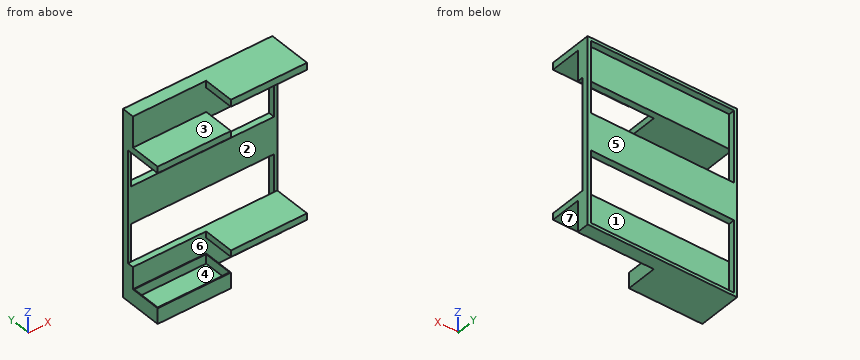
```python
from build123d import *

# Parameters (mm, degrees)
F0_W      = 609.6
F0_H      = 762
F0_W_2    = 584.5253169537
F0_H_2    = 736.8236780167
F1_DEPTH  = 25.4
F2_W      = 584.5253169537
F2_H      = 140.0518767754
F3_DEPTH  = 25.4
F4_W      = 609.6
F4_H      = 152.9776729027
F5_DEPTH  = 25.4
F6_W      = 607.6588928699
F6_H      = 151.1828005314
F7_DEPTH  = 25.4
F8_W      = 310.3615156889
F8_H      = 26.3459533453
F9_DEPTH  = 127
F10_W     = 299.2384843111
F10_H     = 25.4
F11_DEPTH = 127
F12_W     = 299.2384843111
F12_H     = 127
F12_W_2   = 293.7446322758
F12_H_2   = 120.7347996533
F13_DEPTH = 38.1
F14_W     = 299.2384843111
F14_H     = 26.3609342495
F14_W_2   = 310.3615156889
F14_H_2   = 28.4420627674
F15_DEPTH = 127


with BuildPart() as f1:
    # F0 (on Front) → F1 (new body)
    with BuildSketch(Plane.XZ):
        with Locations((5.5615156889, 74.8699506839)):
            Rectangle(F0_W, F0_H)
        with Locations((4.7548860312, 75.109988451)):
            Rectangle(F0_W_2, F0_H_2, mode=Mode.SUBTRACT)
    extrude(amount=F1_DEPTH)

    # F2 (on face) → F3 (join)
    with BuildSketch(Plane.XZ.offset(25.4)):
        with Locations((4.7548860312, 373.4958890716)):
            Rectangle(F2_W, F2_H)
        Polygon((310.3615156889, 455.8699506839), (-299.2384843111, 455.8699506839), (-299.2384843111, 303.4699506839), (-287.5077724457, 303.4699506839), (-287.5077724457, 443.5218274593), (297.017544508, 443.5218274593), (297.017544508, 303.4699506839), (310.3615156889, 303.4699506839), align=None)
    extrude(amount=F3_DEPTH)

    # F4 (on face) → F5 (join)
    with BuildSketch(Plane.XZ.offset(25.4)):
        with Locations((5.5615156889, -229.6412128647)):
            Rectangle(F4_W, F4_H)
    extrude(amount=F5_DEPTH)

    # F6 (on Front) → F7 (join)
    with BuildSketch(Plane.XZ):
        with Locations((5.5615156889, 75.5914002657)):
            Rectangle(F6_W, F6_H)
    extrude(amount=F7_DEPTH)

    # F8 (on face) → F9 (join)
    with BuildSketch(Plane.XZ.offset(50.8)):
        with Locations((155.1807578444, -166.325353086)):
            Rectangle(F8_W, F8_H)
    extrude(amount=F9_DEPTH)

    # F10 (on face) → F11 (join)
    with BuildSketch(Plane.XZ.offset(50.8)):
        with Locations((-149.6192421556, -293.4300493161)):
            Rectangle(F10_W, F10_H)
    extrude(amount=F11_DEPTH)

    # F12 (on face) → F13 (join)
    with BuildSketch(Plane.XY.offset(-280.7300493161)):
        with Locations((-149.6192421556, -114.3)):
            Rectangle(F12_W, F12_H)
        with Locations((-149.3473903975, -113.9315422624)):
            Rectangle(F12_W_2, F12_H_2, mode=Mode.SUBTRACT)
    extrude(amount=F13_DEPTH)

    # F14 (on face) → F15 (join)
    with BuildSketch(Plane.XZ.offset(50.8)):
        with Locations((-149.6192421556, 316.6504178087)):
            Rectangle(F14_W, F14_H)
        with Locations((155.1807578444, 441.6489193003)):
            Rectangle(F14_W_2, F14_H_2)
    extrude(amount=F15_DEPTH)


solid = f1.part
```
Work out the finished part from the listing and answer in its coordinate system (mm). Face numbers are marked on the shaded views. A direction names the side the tool comes from. Give positions to 0.01 mm unless a question says otherwise; leave off trailing zeros. Loops run counter-clockwise (first coordinate to the right, second up) from the corner with the lowest first, then second, coordinate; pieces in that order, holes last. Notation, with made-up numbers: M 26.5,86 L 47.5,86 A14 cw 47.5,106 Z; hole C -33,89 d4. An arc over 180 degrees is marked long. One line per item, written item: value. Start each with the question number.
1. Find section D-D (y = -100.5). Give the vertices of the cut face in (x, z), and give its area (3 significant figures).
2. Find the intervals of material crossed by probe 1 along Z at (x, y) = (126, -36); probe 2 along Z at (x, y) = (23, -59.5); probe 3 along X at (y, z) = (-19.5, 220), in increasing order.
3. Find section C-C (z = -121). Give the vertices of the cut face in (x, y), and give its area (3 significant figures).
4. Each of these flat-tipped pins is pushed along its axis until it touches: P1, Ø4, axis at y = -59.5, z = -175.5, coming from the -X side; P2, Ø8, axis at x = -155.5, z = 375.5, coming from the +Y side; P3, Ø19, axis at y = -116.5, z = -252.5, coming from the +X side; P4, Ø1, axis at x = 174.5, z = 102, coming from the +Y side. Where does it stop, or does it pass through?
5. Find section A-A (x = 33). Give the vertices of the cut face in (y, z).
6. Which of the six approach directions +Z, -Z, +X, -X, +Y, -Y give full straight-line access (tool end or side, diameter ignored) to the marked faces 1, 2, 3 and 4?
7. Find section B-B (y = -15.5). Give the vertices of the cut face in (x, z).
8. Determine the mould class of the marked faces 5, 6 and 7 for opening direction Z: released by +Z, released by -Z, zero draft, split by the parting line, or undercut.
Reported:
1. outline: M -299.24,-306.13 L 0,-306.13 L 0,-242.63 L -2.48,-242.63 L -2.48,-280.73 L -296.22,-280.73 L -296.22,-242.63 L -299.24,-242.63 Z; M -299.24,303.47 L 0,303.47 L 0,329.83 L -299.24,329.83 Z; M 0,-179.5 L 310.36,-179.5 L 310.36,-153.15 L 0,-153.15 Z; M 0,427.43 L 310.36,427.43 L 310.36,455.87 L 0,455.87 Z
1. area: 32,700 mm²
2. probe 1: z = -306.13 to -153.15, 303.47 to 455.87
2. probe 2: z = -179.5 to -153.15, 427.43 to 455.87
2. probe 3: x = -299.24 to -287.51, 297.02 to 310.36
3. outline: M -299.24,-25.4 L -287.51,-25.4 L -287.51,0 L -299.24,0 Z; M 297.02,-25.4 L 310.36,-25.4 L 310.36,0 L 297.02,0 Z
3. area: 637 mm²
4. P1: stops at x = 0
4. P2: stops at y = -25.4
4. P3: stops at x = 0
4. P4: stops at y = 0
5. outline: M -177.8,-179.5 L -50.8,-179.5 L -50.8,-306.13 L 0,-306.13 L 0,-293.3 L -25.4,-293.3 L -25.4,-153.15 L -177.8,-153.15 Z; M -177.8,427.43 L -50.8,427.43 L -50.8,303.47 L -25.4,303.47 L -25.4,443.52 L 0,443.52 L 0,455.87 L -177.8,455.87 Z; M -25.4,0 L 0,0 L 0,151.18 L -25.4,151.18 Z
6. face 1: +Y
6. face 2: +X, -X, -Y
6. face 3: +Z, +X, -X, -Y
6. face 4: none
7. outline: M -299.24,-306.13 L 310.36,-306.13 L 310.36,455.87 L -299.24,455.87 Z; hole M -287.51,-293.3 L 297.02,-293.3 L 297.02,0 L -287.51,0 Z; hole M -287.51,151.18 L 297.02,151.18 L 297.02,443.52 L -287.51,443.52 Z
8. face 5: zero draft
8. face 6: undercut
8. face 7: released by -Z
